Design review of the part built by this model. Coordinates are the model's own, in mm. A direction names the side the tool comes from. Give positions to 0.01 mm unless a question says otherwise; leave off trailing zeros. Loops run counter-clockwise (first coordinate to the right, second up) from the corner with the lowest first, then second, coordinate; pieces in that order, holes last.
from build123d import *

# Parameters (mm, degrees)
PAD002_DEPTH    = 48
POCKET003_DEPTH = 5


with BuildPart() as pad002:
    # Sketch001 → Pad002 (new body)
    with BuildSketch(Plane.XZ):
        with BuildLine():
            Line((-17.5, 6.5), (-14, 6.5))
            ThreePointArc((-13.5, 6), (-13.646447, 6.353553), (-14, 6.5))
            Line((-13.5, 6), (-13.5, 0.5))
            ThreePointArc((-13.5, 0.5), (-13.353553, 0.146447), (-13, 0))
            Line((-13, 0), (13, 0))
            ThreePointArc((13, 0), (13.353553, 0.146447), (13.5, 0.5))
            Line((13.5, 0.5), (13.5, 6))
            ThreePointArc((14, 6.5), (13.646447, 6.353553), (13.5, 6))
            Line((14, 6.5), (17.5, 6.5))
            Line((17.5, 6.5), (17.5, 7.5))
            Line((17.5, 7.5), (13, 7.5))
            ThreePointArc((13, 7.5), (12.646447, 7.353553), (12.5, 7))
            Line((12.5, 7), (12.5, 1.5))
            ThreePointArc((12, 1), (12.353553, 1.146447), (12.5, 1.5))
            Line((12, 1), (-12, 1))
            ThreePointArc((-12.5, 1.5), (-12.353553, 1.146447), (-12, 1))
            Line((-12.5, 1.5), (-12.5, 7))
            ThreePointArc((-12.5, 7), (-12.646447, 7.353553), (-13, 7.5))
            Line((-13, 7.5), (-17.5, 7.5))
            Line((-17.5, 7.5), (-17.5, 6.5))
        make_face()
    extrude(amount=PAD002_DEPTH)


with BuildPart() as common:
    # Pocket003 base: copy of Pad002
    add(pad002.part)

    # Sketch002 (on Face19 of Pad002) → Pocket003 (cut)
    with BuildSketch(Plane(origin=(0, 0, 1), x_dir=(-1, 0, 0), z_dir=(0, 0, 1))):
        with BuildLine():
            ThreePointArc((-2.55, 33), (0, 30.45), (2.55, 33))
            Line((2.55, 33), (2.55, 43))
            ThreePointArc((2.55, 43), (0, 45.55), (-2.55, 43))
            Line((-2.55, 33), (-2.55, 43))
        make_face()
        with BuildLine():
            ThreePointArc((-2.55, 8), (0, 5.45), (2.55, 8))
            Line((2.55, 8), (2.55, 18))
            ThreePointArc((2.55, 18), (0, 20.55), (-2.55, 18))
            Line((-2.55, 8), (-2.55, 18))
        make_face()
    extrude(amount=-POCKET003_DEPTH, mode=Mode.SUBTRACT)

    # Common: intersect Pad002
    add(pad002.part, mode=Mode.INTERSECT)


solid = common.part
Q1. Wall thickness on line 1 (X direction, y = -32, z = 4); line 2 (Z direction, x = -15, y = -26.5); line 3 (Z direction, x = 11, y = -25.5): over which ranges is each line inside the solid? List them lowest first.
Results:
line 1: x = -13.5 to -12.5, 12.5 to 13.5
line 2: z = 6.5 to 7.5
line 3: z = 0 to 1
Q2. Tool access review of faces 1 (the face through (16, -24, 6.5)), 2 (the face through (-2.55, -37.9, 0.5)), 3 (the face through (0, -24, 0)), 4 (the face through (12.5, -24, 4)), 5 (the face through (-16, -24, 6.5)): name each direction out of +Z, -Z, +X, -X, +Y, -Y from which nothing blocks a thin tool from reaching the whole face with its end or side.
Results:
face 1: -Z, +X, +Y, -Y
face 2: +Z, -Z
face 3: -Z, +X, -X, +Y, -Y
face 4: +Z, +Y, -Y
face 5: -Z, -X, +Y, -Y
Q3. Take a section at C-C (y = -10.5). Give the boundary of the cut face in (x, z), plus the area to 3 significant figures.
Results:
outline: (-17.5, 6.5) - (-14, 6.5) arc R0.5 cw to (-13.5, 6) - (-13.5, 0.5) arc R0.5 ccw to (-13, 0) - (-2.55, 0) - (-2.55, 1) - (-12, 1) arc R0.5 cw to (-12.5, 1.5) - (-12.5, 7) arc R0.5 ccw to (-13, 7.5) - (-17.5, 7.5) - close; (2.55, 0) - (13, 0) arc R0.5 ccw to (13.5, 0.5) - (13.5, 6) arc R0.5 cw to (14, 6.5) - (17.5, 6.5) - (17.5, 7.5) - (13, 7.5) arc R0.5 ccw to (12.5, 7) - (12.5, 1.5) arc R0.5 cw to (12, 1) - (2.55, 1) - close
area: 42.9 mm2
Q4. Insertion check: pin 1 (10 mm diameter, centred on x = 5, y = -41.5, fed in from +Z); pin 2 (0.5 mm diameter, centred on y = -38.5, z = 0.5, fed in from -X); pin 3 (3 mm diameter, centred on x = -15.5, y = -32.5, fed in from -Z). Each pin has a flat end and moves straight along its axis. Give the tip position at first contact, or say it passes through.
Results:
pin 1: stops at z = 1
pin 2: stops at x = -13.5
pin 3: stops at z = 6.5
Q5. Take a section at D-D (y = -24). Give the boundary of the cut face in (x, z), plus the area to 3 significant figures.
Results:
outline: (-17.5, 6.5) - (-14, 6.5) arc R0.5 cw to (-13.5, 6) - (-13.5, 0.5) arc R0.5 ccw to (-13, 0) - (13, 0) arc R0.5 ccw to (13.5, 0.5) - (13.5, 6) arc R0.5 cw to (14, 6.5) - (17.5, 6.5) - (17.5, 7.5) - (13, 7.5) arc R0.5 ccw to (12.5, 7) - (12.5, 1.5) arc R0.5 cw to (12, 1) - (-12, 1) arc R0.5 cw to (-12.5, 1.5) - (-12.5, 7) arc R0.5 ccw to (-13, 7.5) - (-17.5, 7.5) - close
area: 48.0 mm2
Q6. Take a section at A-A (z = 3.5). Give the boundary of the cut face in (x, y).
Results:
outline: (-13.5, -48) - (-12.5, -48) - (-12.5, 0) - (-13.5, 0) - close; (12.5, -48) - (13.5, -48) - (13.5, 0) - (12.5, 0) - close
Q7. Take a section at B-B (x = 0). Give the boundary of the cut face in (y, z).
Results:
outline: (-48, 0) - (-45.55, 0) - (-45.55, 1) - (-48, 1) - close; (-30.45, 0) - (-20.55, 0) - (-20.55, 1) - (-30.45, 1) - close; (-5.45, 0) - (0, 0) - (0, 1) - (-5.45, 1) - close
